Check sheet for the drawn part. Datum: minimum x, y, z corner. Units: mm. A direction names the side the tool comes from. Round coordinates to 2 decimals unless told otherwise and drop trailing zeros. Order: outer loops, then holes, each group sorted by start corner. A loop starts at its lowest first (then second) coordinate and runs counter-clockwise, first axis right, second up.
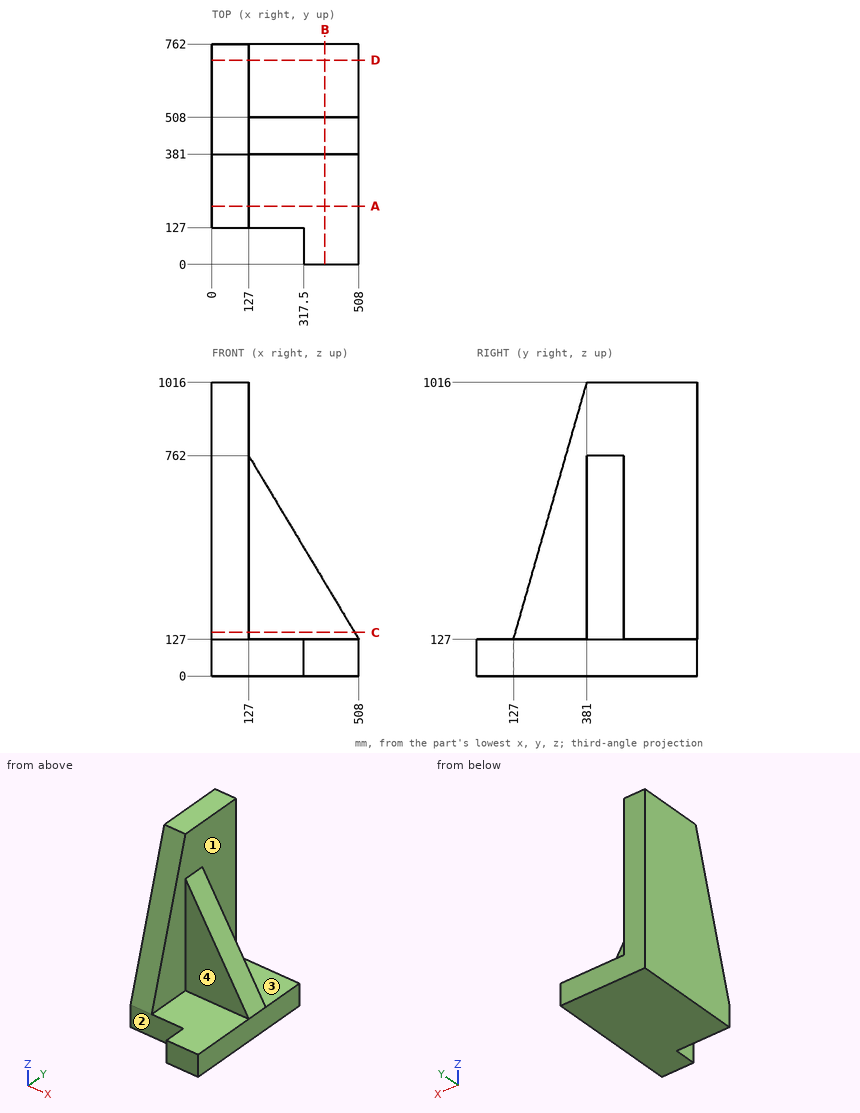
(1) Set-up check for the marked faces 1, 2, 3 and 4: record each of +Z, -Z, +X, -X, +Y, -Y from which the full face is reachable in a straight line by a thin tool's end or side.
Returned:
face 1: +Z, +X
face 2: +Z, -Z, -X, -Y
face 3: +Z, +X, +Y
face 4: +Z, +X, -Y
(2) Material ranges on line 1 (X direction, y = 716, z = 708.5); line 2 (Y direction, x = 199, z = 266), recorded low to high.
Returned:
line 1: x = 0 to 127
line 2: y = 381 to 508
(3) Sectioned sample at C-C, the plane z = 151. Record the cut outline in (x, y), and give its area (3 significant figures).
Returned:
outline: (0, 133.86) - (127, 133.86) - (127, 381) - (493.6, 381) - (493.6, 508) - (127, 508) - (127, 762) - (0, 762) - close
area: 126,000 mm2
(4) Sectioned sample at B-B, the plane x = 391. Record the cut outline in (y, z), and give its area (3 significant figures).
Returned:
outline: (0, 0) - (762, 0) - (762, 127) - (508, 127) - (508, 322) - (381, 322) - (381, 127) - (0, 127) - close
area: 122,000 mm2
(5) Depth check by flat-ended pin: P1, Ø4, axis at y = 378, z = 451, coming from the +X side; P2, Ø4, axis at x = 400, y = 406, coming from the -Z side; P3, Ø10, axis at x = 224, z = 141, coming from the +Y side; P4, Ø10, axis at x = 68, z = 583, coming from the -Y side. Enter the tip coordinate at first touch or a pass-through.
Returned:
P1: stops at x = 127
P2: stops at z = 0
P3: stops at y = 508
P4: stops at y = 255.86
(6) Sectioned sample at D-D, the plane y = 706. Record the cut outline in (x, z), and give its area (3 significant figures).
Returned:
outline: (0, 0) - (508, 0) - (508, 127) - (127, 127) - (127, 1016) - (0, 1016) - close
area: 177,000 mm2
(7) Sectioned sample at A-A, the plane y = 201. Record the cut outline in (x, z), and give its area (3 significant figures).
Returned:
outline: (0, 0) - (508, 0) - (508, 127) - (127, 127) - (127, 386) - (0, 386) - close
area: 97,400 mm2
